Work out the finished part from the listing and answer in its coordinate system (mm). A direction names the side the tool comes from. Coordinates: 2 decimals unless noted, no trailing zeros. Order: outer loops, then holes, each group sorted by start corner. A loop starts at its lowest first (then second) coordinate and runs counter-clockwise, first axis right, second up. Notation, with made-up numbers: M 51,-4 L 107,-4 A22 cw 107,19 Z; hole C 16.5,27 d2. An arc over 180 degrees is marked long. Answer in a Markdown table with one row per item. Add a question column.
Item 1: The part is cut by section D-D (z = 2.5). Write down the section's boundary in (x, y), then the cut area to 3 significant figures.
Item 2: Flat-ended cylindrical pins translate along their axes: pin 1 Ø4 at (y, z) = (-1, 5.5) entering from +X; pin 2 Ø1 at (x, y) = (-4, 6) entering from -Z; pin 3 Ø1 at (x, z) = (-4, 3.5) entering from +Y. Find the tip coordinate at first contact, or state that the pin passes through.
Item 3: The mould has two halves that part along X. Classify faces 1 (the face through (-1.73, -7.81, 1.09)), 2 (the face through (-3, 0, 4)), 3 (the face through (1.6, -3.3, 0)): released by +X, released by -X, zero draft, split by the parting line, or undercut.
Item 4: The part is cut by section A-A (y = 0). Write down the section's boundary in (x, z).
Item 5: Which of the six approach directions +Z, -Z, +X, -X, +Y, -Y give full straight-line access (tool end or side, diameter ignored) to faces 4 (the face through (2.3, -2.3, 7.2)), 5 (the face through (4.896, -2.03, 4.665))?
Item 6: The part is cut by section C-C (z = 1.5). Write down the section's boundary in (x, y), then the cut area to 3 significant figures.
Item 7: Consider line 1 (Y direction, x = 0, z = 3.25); line 2 (Z direction, x = 6.5, y = -4); line 3 (Y direction, x = 2.5, z = 1). Determine where each line is inside the solid, lowest interval first. Write a range as from..to.
from build123d import *

# Parameters (mm, degrees)
F0_R     = 5.3
F0_R_2   = 3
F1_DEPTH = 7.2
F0_R_3   = 8
F2_DEPTH = 2.2
F3_SIZE  = 0.5
F4_SIZE  = 0.3
F5_SIZE  = 0.3


with BuildPart() as f1:
    # F0 (on Top) → F1 (new body)
    with BuildSketch(Plane.XY):
        Circle(F0_R)
        Circle(F0_R_2, mode=Mode.SUBTRACT)
    extrude(amount=F1_DEPTH)

    # F0 (on Top) → F2 (join)
    with BuildSketch(Plane.XY):
        Circle(F0_R_3)
        Circle(F0_R, mode=Mode.SUBTRACT)
    extrude(amount=F2_DEPTH)

    # F3
    f3_edges = [f1.edges().sort_by_distance(p)[0] for p in [
        (-3, 0, 0),
    ]]
    chamfer(f3_edges, length=F3_SIZE)

    # F4
    f4_edges = [f1.edges().sort_by_distance(p)[0] for p in [
        (-8, 0, 2.2),
    ]]
    chamfer(f4_edges, length=F4_SIZE)

    # F5
    f5_edges = [f1.edges().sort_by_distance(p)[0] for p in [
        (-8, 0, 0),
    ]]
    chamfer(f5_edges, length=F5_SIZE)


solid = f1.part
Reply:
| question | item | result |
|---|---|---|
| 1 | outline | C 0,0 d10.6; hole C 0,0 d6 |
| 1 | area | 60.0 mm2 |
| 2 | pin 1 | stops at x = 5.3 |
| 2 | pin 2 | stops at z = 0 |
| 2 | pin 3 | stops at y = 3.98 |
| 3 | face 1 | split by the parting line |
| 3 | face 2 | undercut |
| 3 | face 3 | zero draft |
| 4 | outline | M -8,0.3 L -7.7,0 L -3.5,0 L -3,0.5 L -3,7.2 L -5.3,7.2 L -5.3,2.2 L -7.7,2.2 L -8,1.9 Z; M 3,0.5 L 3.5,0 L 7.7,0 L 8,0.3 L 8,1.9 L 7.7,2.2 L 5.3,2.2 L 5.3,7.2 L 3,7.2 Z |
| 5 | face 4 | +Z, +X, -X, +Y, -Y |
| 5 | face 5 | +Z |
| 6 | outline | C 0,0 d16; hole C 0,0 d6 |
| 6 | area | 173 mm2 |
| 7 | line 1 | y = -5.3..-3, 3..5.3 |
| 7 | line 2 | z = 0..2.2 |
| 7 | line 3 | y = -7.6..-1.66, 1.66..7.6 |
